from build123d import *

# Parameters (mm, degrees)
SKETCH13_W        = 1.25
SKETCH13_H        = 11
CIRPATTERN1_COUNT = 4


with BuildPart() as part:
    # Sketch11 → Revolve1 (revolve)
    with BuildSketch(Plane.XY):
        Polygon((8, 40), (2.5, 40), (2.5, 0), (11, 0), (11, 4), (8, 7), (8, 35), align=None)
    revolve(axis=Axis((0, 0, 0), (0, 1, 0)))

    # Sketch13 → M3x0.5 Tapped Hole1 (revolve, cut)
    with BuildSketch(Plane(origin=(0, 2, 0), x_dir=(0, 0, -1), z_dir=(0, 1, 0))):
        with Locations((0.625, 5.5)):
            Rectangle(SKETCH13_W, SKETCH13_H)
    m3x0_5_tapped_hole1 = revolve(axis=Axis((6.35, 2, 0), (-1, 0, 0)), mode=Mode.SUBTRACT)

    # CirPattern1: M3x0.5 Tapped Hole1 ×4 about axis
    cirpattern1_axis = Axis((0, 0, 0), (0, -1, 0))
    for i in range(1, CIRPATTERN1_COUNT):
        add(m3x0_5_tapped_hole1.rotate(cirpattern1_axis, i * 360 / CIRPATTERN1_COUNT), mode=Mode.SUBTRACT)


solid = part.part
Verification items for the finished model (mm, model axes). Give positions to 0.01 mm unless a question says otherwise; leave off trailing zeros. Loops run counter-clockwise (first coordinate to the right, second up) from the corner with the lowest first, then second, coordinate; pieces in that order, holes last. Notation, with made-up numbers: (74.25, 4) - (115.25, 4) arc R14 ccw to (115.25, 16) - close; hole circle Ø10 at (-9.75, 50.25). An arc over 180 degrees is marked (long way). Write item = value, one per line. Start each with the question number.
Q1. Mould release check, pull along X, two halves, no side actions. Record for faces 1 (the face through (-1.73, 23.73, 7.81)), 2 (the face through (-6.64, 0.76, 0.16)), 3 (the face through (-0.16, 0.76, -6.64)): released by +X, released by -X, zero draft, split by the parting line, or undercut.
Q2. Thickness scan on line 1 (Y direction, x = 0, z = 6); line 2 (X direction, y = 13.5, z = 0). Record the ranges inside material, lowest first.
Q3. Cross-section at C-C, the plane y = 2. Enter the section's corners in (x, z), and give its area (3 significant figures).
Q4. Cross-section at A-A, the plane z = 0. Enter the section's corners in (x, y), and give its area (4 significant figures).
Q5. Cross-section at B-B, the plane x = 0. Enter the section's corners in (y, z).
Q6. Depth check by flat-ended pin: P1, Ø4, axis at y = 23, z = 1, coming from the +X side; P2, Ø8, axis at y = 16.5, z = -4.5, coming from the -X side; P3, Ø6, axis at y = 5.5, z = 7, coming from the -X side; P4, Ø3, axis at x = 0, z = 0, coming from the +Y side. Enter the tip coordinate at first touch or a pass-through.
Q7. Cross-section at D-D, the plane y = 25.5. Enter the section's corners in (x, z).
Answer key:
q1.face_1 = split by the parting line
q1.face_2 = zero draft
q1.face_3 = undercut
q2.line_1 = 0 to 0.75, 3.25 to 40
q2.line_2 = -8 to -2.5, 2.5 to 8
q3.outline = (-10.93, -1.25) arc R11 ccw to (-1.25, -10.93) - (-1.25, -2.17) arc R2.5 cw to (-2.17, -1.25) - close; (-10.93, 1.25) - (-2.17, 1.25) arc R2.5 cw to (-1.25, 2.17) - (-1.25, 10.93) arc R11 ccw to start; (1.25, -10.93) arc R11 ccw to (10.93, -1.25) - (2.17, -1.25) arc R2.5 cw to (1.25, -2.17) - close; (1.25, 2.17) arc R2.5 cw to (2.17, 1.25) - (10.93, 1.25) arc R11 ccw to (1.25, 10.93) - close
q3.area = 275 mm^2
q4.outline = (-11, 0) - (-2.5, 0) - (-2.5, 0.75) - (-11, 0.75) - close; (-11, 3.25) - (-2.5, 3.25) - (-2.5, 40) - (-8, 40) - (-8, 7) - (-11, 4) - close; (2.5, 0) - (11, 0) - (11, 0.75) - (2.5, 0.75) - close; (2.5, 3.25) - (11, 3.25) - (11, 4) - (8, 7) - (8, 40) - (2.5, 40) - close
q4.area = 430.5 mm^2
q5.outline = (0, -11) - (0.75, -11) - (0.75, -2.5) - (0, -2.5) - close; (0, 2.5) - (0.75, 2.5) - (0.75, 11) - (0, 11) - close; (3.25, -11) - (4, -11) - (7, -8) - (40, -8) - (40, -2.5) - (3.25, -2.5) - close; (3.25, 2.5) - (40, 2.5) - (40, 8) - (7, 8) - (4, 11) - (3.25, 11) - close
q6.P1 = 8
q6.P2 = -7.98
q6.P3 = -10.08
q6.P4 = through
q7.outline = circle Ø16 at (0, 0); hole circle Ø5 at (0, 0)
